Source: CAD feature listing. Evaluate the final solid. Frame: model axes, mm. Round coordinates to 2 decimals unless told otherwise and drop trailing zeros. Write each loop counter-clockwise with the first axis right and the second up, starting at its lowest first coordinate (ties: lowest second). Pieces come first, ordered by that corner, then holes. Notation, with made-up numbers: M -19.5,89 L 20.5,89 A22 cw 20.5,125 Z; hole C 63,58.25 d9. An arc over 180 degrees is marked long. Answer in a Markdown table with one row per item.
from build123d import *

# Parameters (mm, degrees)
SKETCH1_W           = 10
SKETCH1_H           = 10
BOSS_EXTRUDE2_DEPTH = 200
SKETCH3_W           = 8
SKETCH3_H           = 8
CUT_EXTRUDE1_DEPTH  = 200
SKETCH4_R           = 3.575
SKETCH4_R_2         = 2.25
SKETCH4_R_3         = 2.2
CUT_EXTRUDE2_DEPTH  = 201.31225624
FILLET1_R           = 1


with BuildPart() as part:
    # Sketch1 → Boss-Extrude2 (new body)
    with BuildSketch(Plane(origin=(0, 0, 0), x_dir=(1, 0, 0), z_dir=(0, 1, 0))):
        Rectangle(SKETCH1_W, SKETCH1_H)
    extrude(amount=BOSS_EXTRUDE2_DEPTH)

    # Sketch3 → Cut-Extrude1 (cut)
    with BuildSketch(Plane(origin=(0, 200, 0), x_dir=(1, 0, 0), z_dir=(0, 1, 0))):
        Rectangle(SKETCH3_W, SKETCH3_H)
    extrude(amount=-CUT_EXTRUDE1_DEPTH, mode=Mode.SUBTRACT)

    # Sketch4 → Cut-Extrude2 (cut, through all)
    with BuildSketch(Plane(origin=(5, 0, 0), x_dir=(0, 0, -1), z_dir=(1, 0, 0))):
        with Locations((0, 100)):
            Circle(SKETCH4_R)
        with Locations((0, 190)):
            Circle(SKETCH4_R_2)
        with Locations((0, 10)):
            Circle(SKETCH4_R_3)
    extrude(amount=-CUT_EXTRUDE2_DEPTH, mode=Mode.SUBTRACT)

    # Fillet1
    fillet1_edges = [part.edges().sort_by_distance(p)[0] for p in [
        (4, 200, 0),
        (0, 200, -4),
        (-4, 200, 0),
        (0, 200, 4),
        (0, 0, 5),
        (-5, 0, 0),
        (0, 0, -5),
        (5, 0, 0),
    ]]
    fillet(fillet1_edges, radius=FILLET1_R - 0.0001)  # a hair under: the kernel refuses the full size


solid = part.part
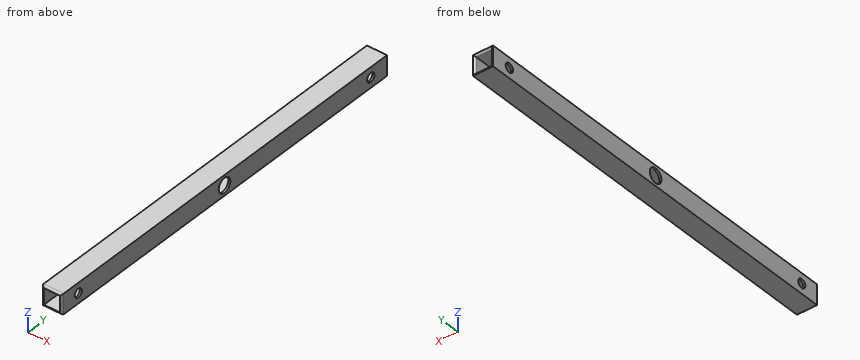
Q1. Section C-C (y = 20.5). Return loops of the section in (x, z), and give its area (3 significant figures).
Solutions:
| item | result |
|---|---|
| outline | M -5,-5 L 5,-5 L 5,5 L -5,5 Z; hole M -4,-4 L 4,-4 L 4,4 L -4,4 Z |
| area | 36.0 mm2 |
Q2. Material intervals for probe 1 along Z at (x, y) = (-0.5, 165); probe 2 along Y at (x, z) = (4.25, 0.75), sorted ascending.
Solutions:
| item | result |
|---|---|
| probe 1 | z = -5 to -4, 4 to 5 |
| probe 2 | y = 0.03 to 7.93, 12.07 to 96.5, 103.5 to 187.88, 192.12 to 199.66 |
Q3. Section D-D (z = 0). State how many separate pieces and enclosed holes the cut face has, and give its area (3 significant figures).
Solutions:
| item | result |
|---|---|
| separate pieces | 8 |
| enclosed holes | 0 |
| area | 367 mm2 |
Q4. Section A-A (y = 190). Return loops of the section in (x, z), and give its area (3 significant figures).
Solutions:
| item | result |
|---|---|
| outline | M -5,-5 L 5,-5 L 5,-2.25 L 4,-2.25 L 4,-4 L -4,-4 L -4,-2.25 L -5,-2.25 Z; M -5,2.25 L -4,2.25 L -4,4 L 4,4 L 4,2.25 L 5,2.25 L 5,5 L -5,5 Z |
| area | 27.0 mm2 |
